The figure shows three views and two pictorial views of one solid part (mm, origin at its lowest corner). Answer the questions. A direction names the side the tool comes from. Round coordinates to 2 decimals unless told otherwise and drop trailing zeros. Order: outer loops, then holes, each group sorted by start corner. A loop starts at its lowest first (then second) coordinate and runs counter-clockwise, first axis right, second up. Notation, with made-up numbers: M 39.25,81.5 L 98.25,81.5 A5 cw 98.25,86.5 Z; hole C 9.5,16 d1. An arc over 180 degrees is marked long. Answer as CSV lines item,"result".
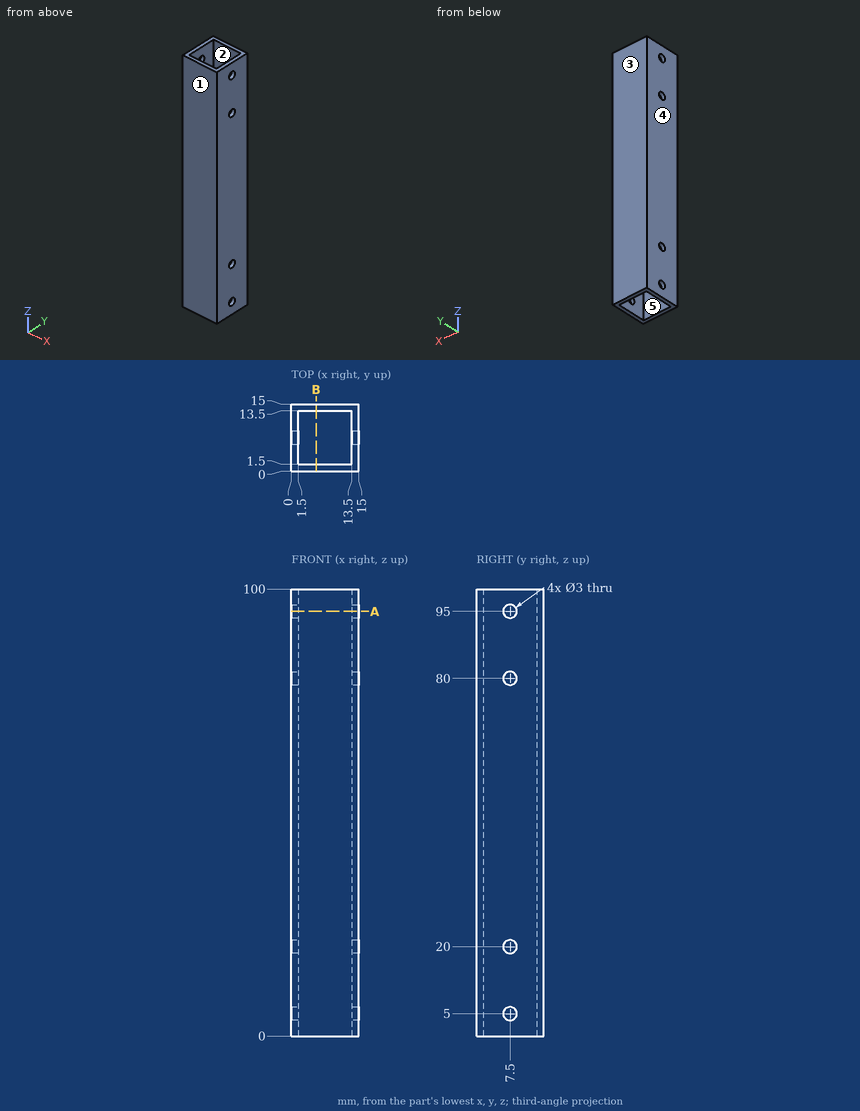
Item 1: A cutting plane is placed at B-B, the plane x = 5.5. Determine the outline of the cut face in (y, z).
Ans:
outline,"M 0,0 L 1.5,0 L 1.5,100 L 0,100 Z; M 13.5,0 L 15,0 L 15,100 L 13.5,100 Z"
Item 2: Find the intervals of material crossed by probe 1 along Y at (x, z) = (1.05, 95); probe 2 along X at (y, z) = (12, 62.5), in increasing order. Write a range as [from, to].
Ans:
probe 1,"[0, 6], [9, 15]"
probe 2,"[0, 1.5], [13.5, 15]"
Item 3: A tool of negligible diameter and unlimited length cuts with its end or side. For the marked faces 1 and 2, from which of +Z, -Z, +X, -X, +Y, -Y can it reach the whole face along a straight path? Write none if from no direction.
Ans:
face 1,"+Z, -Z, +X, -X, -Y"
face 2,"+Z, -Z"
Item 4: A flat-ended cylindrical pin translates along its axis: pin 1 (5 mm diameter, centred on x = 12.5, y = 9.5, fed in from -Z). Find the tip coordinate at first contact, or state that the pin passes through.
Ans:
pin 1,"z = 0"
Item 5: A cutting plane is placed at A-A, the plane z = 95. Determine the outline of the cut face in (x, y), and give its area (3 significant figures).
Ans:
outline,"M 0,0 L 15,0 L 15,6 L 13.5,6 L 13.5,1.5 L 1.5,1.5 L 1.5,6 L 0,6 Z; M 0,9 L 1.5,9 L 1.5,13.5 L 13.5,13.5 L 13.5,9 L 15,9 L 15,15 L 0,15 Z"
area,"72.0 mm2"
Item 6: Determine the mould class of the marked faces 3, 4 and 5 for opening direction Y: +Y half, -Y half, draft (parallel to the pull), parting line (faces both ways), or undercut.
Ans:
face 3,"+Y half"
face 4,"draft"
face 5,"undercut"
